from build123d import *

# Parameters (mm, degrees)
SKETCH1_W           = 55
SKETCH1_H           = 25
SKETCH1_R           = 2.435064935
BOSS_EXTRUDE1_DEPTH = 10
SKETCH2_W           = 27
SKETCH2_H           = 25
BOSS_EXTRUDE2_DEPTH = 30
SKETCH3_W           = 27
SKETCH3_H           = 25
BOSS_EXTRUDE3_DEPTH = 30
SKETCH4_R           = 5
CUT_EXTRUDE1_DEPTH  = 20


with BuildPart() as part:
    # Sketch1 → Boss-Extrude1 (new body)
    with BuildSketch(Plane.XY):
        with Locations((27.5, 12.5)):
            Rectangle(SKETCH1_W, SKETCH1_H)
        with Locations((52.5, 12.5)):
            Circle(SKETCH1_R, mode=Mode.SUBTRACT)
        with Locations((2.5, 12.5)):
            Circle(SKETCH1_R, mode=Mode.SUBTRACT)
    extrude(amount=BOSS_EXTRUDE1_DEPTH)

    # Sketch2 → Boss-Extrude2 (add)
    with BuildSketch(Plane.XY.offset(10)):
        with Locations((27.5, 12.5)):
            Rectangle(SKETCH2_W, SKETCH2_H)
    extrude(amount=BOSS_EXTRUDE2_DEPTH)

    # Sketch3 → Boss-Extrude3 (add)
    with BuildSketch(Plane.XZ):
        with Locations((27.5, 27.5)):
            Rectangle(SKETCH3_W, SKETCH3_H)
    extrude(amount=-BOSS_EXTRUDE3_DEPTH)

    # Sketch4 → Cut-Extrude1 (cut)
    with BuildSketch(Plane.XY.offset(40)):
        with Locations((22.7215485, 15.612504219)):
            Circle(SKETCH4_R)
        with Locations((35.41615295, 17.248010158)):
            Circle(SKETCH4_R)
    extrude(amount=-CUT_EXTRUDE1_DEPTH, mode=Mode.SUBTRACT)


solid = part.part
The model under review builds one solid part; all positions refer to its coordinate system, in mm. A direction names the side the tool comes from. Coordinates: 2 decimals unless noted, no trailing zeros. Loops run counter-clockwise (first coordinate to the right, second up) from the corner with the lowest first, then second, coordinate; pieces in that order, holes last.
(1) Insertion check: P1, Ø7.5, axis at x = 37.5, z = 4, coming from the +Y side; P2, Ø1, axis at y = 22.5, z = 26, coming from the -X side; P3, Ø1, axis at y = 8.5, z = 24, coming from the +X side; P4, Ø3, axis at x = 2.5, y = 12.5, coming from the +Z side. Each pin has a flat end and moves straight along its axis. Give the tip position at first contact, or say it passes through.
Determined:
P1: stops at y = 25
P2: stops at x = 14
P3: stops at x = 41
P4: passes through
(2) Tool access review of faces 1 (the cylindrical face through (25.41, 19.83, 30.14)), 2 (the flat face through (41, 15, 25)), 3 (the flat face through (7, 13, 10)): name each direction out of +Z, -Z, +X, -X, +Y, -Y from which nothing blocks a thin tool from reaching the whole face with its end or side.
Determined:
face 1: +Z
face 2: +Z, +X, +Y, -Y
face 3: +Z, -X, +Y, -Y
(3) Consider section A-A, the plane x = 52.5. Give the boundary of the cut face in (y, z), plus the area to 3 significant figures.
Determined:
outline: (0, 0) - (10.06, 0) - (10.06, 10) - (0, 10) - close; (14.94, 0) - (25, 0) - (25, 10) - (14.94, 10) - close
area: 201 mm2
(4) Consider section B-B, the plane z = 5. Give the boundary of the cut face in (x, y).
Determined:
outline: (0, 0) - (55, 0) - (55, 25) - (0, 25) - close; hole circle Ø4.87 at (2.5, 12.5); hole circle Ø4.87 at (52.5, 12.5)
(5) Wall thickness on L1, parallel to Y at x = 52.5, z = 3; L2, parallel to X at y = 17, z = 21; L3, parallel to X at y = 9.75, z = 28.5: over which ranges is each line inside the solid? List them lowest first.
Determined:
L1: y = 0 to 10.06, 14.94 to 25
L2: x = 14 to 17.92, 27.53 to 30.42, 40.41 to 41
L3: x = 14 to 41
(6) Consider section C-C, the plane y = 14. Give the boundary of the cut face in (x, z).
Determined:
outline: (0, 0) - (0.58, 0) - (0.58, 10) - (0, 10) - close; (4.42, 0) - (50.58, 0) - (50.58, 10) - (41, 10) - (41, 40) - (39.22, 40) - (39.22, 20) - (31.61, 20) - (31.61, 40) - (27.45, 40) - (27.45, 20) - (17.99, 20) - (17.99, 40) - (14, 40) - (14, 10) - (4.42, 10) - close; (54.42, 0) - (55, 0) - (55, 10) - (54.42, 10) - close
(7) Consider section D-D, the plane y = 6. Give the boundary of the cut face in (x, z).
Determined:
outline: (0, 0) - (55, 0) - (55, 10) - (41, 10) - (41, 40) - (14, 40) - (14, 10) - (0, 10) - close
(8) Draft analysis for pull direction Y (two halves, no side actions). For faces 4 (the flat face through (27, 25, 6)), 5 (the flat face through (48, 13, 10)), 6 (the flat face through (27, 0, 15)), 7 (the flat face through (35, 17, 20)), state which applies: +Y half, -Y half, draft (parallel to the pull), parting line (faces both ways), or undercut.
Determined:
face 4: +Y half
face 5: draft
face 6: -Y half
face 7: undercut
